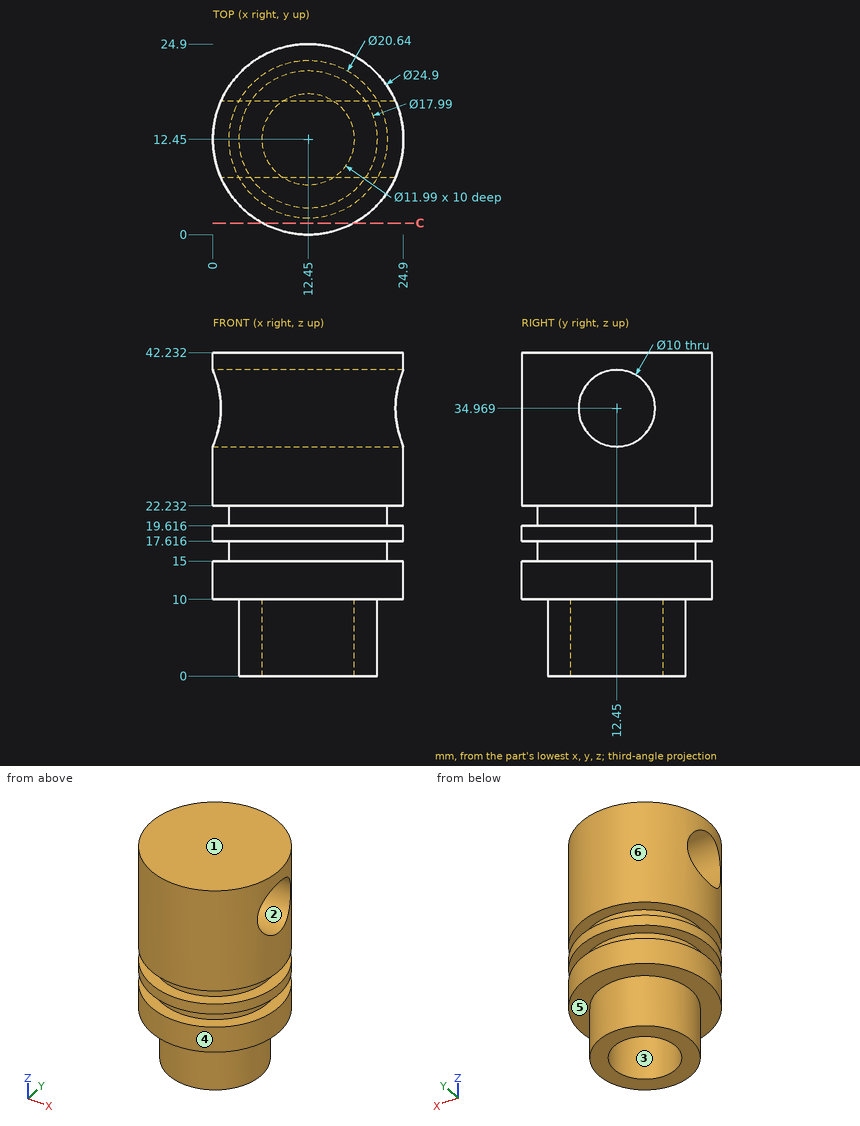
Geometry check sheet. Reference: drawing and pictorial views, mm from the part's lowest x, y, z. A direction names the side the tool comes from. Coordinates: 2 decimals unless noted, no trailing zeros. Order: outer loops, then holes, each group sorted by start corner. A loop starts at its lowest first (then second) coordinate and runs counter-clockwise, first axis right, second up.
Item 1: Mould release check, pull along Y, two halves, no side actions. Record for the marked faces 1, 2, 3 and 4: released by +Y, released by -Y, zero draft, split by the parting line, or undercut.
Item 2: Depth check by flat-ended pin: pin 1 (6 mm diameter, centred on y = 12.45, z = 34.97, fed in from -X); pin 2 (1 mm diameter, centred on x = 10, z = 13, fed in from +Y); pin 3 (1.5 mm diameter, centred on x = 16, y = 13.5, fed in from -Z); pin 4 (3 mm diameter, centred on x = 17, z = 13.5, fed in from -Y). Enter the tip coordinate at first touch or a pass-through.
Item 3: Scan lines: line 1 along Z through (x, y) = (11.5, 23.5); line 2 along X through (y, z) = (12.75, 9.5); line 3 along Z through (x, y) = (3.5, 12). Record each from-to range of solid material in increasing order.
Item 4: Tool access check on the marked faces 5 and 6. Record the directions out of +Z, -Z, +X, -X, +Y, -Y that give a thin tool (end or side, any length) a straight path to the whole face; none if there is none.
Item 5: Section check C-C (y = 1.5). Enter the section's corners in (x, z) (1 decimal), plus the area to 3 significant figures.
Check sheet entries:
1. face 1: zero draft
1. face 2: undercut
1. face 3: undercut
1. face 4: split by the parting line
2. pin 1: passes through
2. pin 2: stops at y = 24.75
2. pin 3: stops at z = 10
2. pin 4: stops at y = 0.38
3. line 1: z = 10 to 15, 17.62 to 19.62, 22.23 to 42.23
3. line 2: x = 3.46 to 6.46, 18.44 to 21.44
3. line 3: z = 0 to 29.99, 39.95 to 42.23
4. face 5: -Z
4. face 6: +Z, -Z
5. outline: (6.5, 10) - (18.4, 10) - (18.4, 15) - (6.5, 15) - close; (6.5, 17.6) - (18.4, 17.6) - (18.4, 19.6) - (6.5, 19.6) - close; (6.5, 22.2) - (18.4, 22.2) - (18.4, 42.2) - (6.5, 42.2) - close
5. area: 320 mm2
